from build123d import *

# Parameters (mm, degrees)
SKETCH021_R      = 1.65
EXTRUDE021_DEPTH = 5
EXTRUDE001_DEPTH = 4
FILLET003_R      = 0.5
BOX005_W         = 48
BOX005_H         = 47
BOX005_DEPTH     = 10
EXTRUDE037_DEPTH = 6
SKETCH038_W      = 10
SKETCH038_H      = 14.5
SKETCH038_R      = 1.25
EXTRUDE038_DEPTH = 4
SKETCH039_W      = 5
SKETCH039_H      = 16
SKETCH039_R      = 1.65
EXTRUDE039_DEPTH = 5
EXTRUDE040_DEPTH = 7
SKETCH020_R      = 1.65
SKETCH020_R_2    = 1.25
SKETCH020_W      = 45
SKETCH020_H      = 10
EXTRUDE036_DEPTH = 4


with BuildPart() as gpshold:
    # Sketch021 → Extrude021 (new body)
    with BuildSketch(Plane.XZ):
        Polygon((65, 28.5), (71, 28.5), (71, 2.5), (65, 2.5), (65, 9), (67, 9), (67, 22), (65, 22), align=None)
        with Locations((67.85, 25.7)):
            Circle(SKETCH021_R, mode=Mode.SUBTRACT)
        with Locations((67.85, 5.4)):
            Circle(SKETCH021_R, mode=Mode.SUBTRACT)
    extrude(amount=EXTRUDE021_DEPTH)


with BuildPart() as gpshold_1:
    # Extrude021 placement: moved
    add(gpshold.part.moved(Location((0, 78.75, 0))))


with BuildPart() as obj1:
    # Sketch001 → Extrude001 (new body)
    with BuildSketch(Plane.XY):
        with BuildLine():
            Line((19.03, 74.44), (19.03, 77.44))
            Line((19.03, 77.44), (13.53, 77.44))
            Line((13.53, 71.94), (13.53, 77.44))
            Line((16.53, 71.94), (13.53, 71.94))
            ThreePointArc((16.53, 71.94), (18.297767, 72.672233), (19.03, 74.44))
        make_face()
        with BuildLine():
            Line((60.53, 34.86), (55.03, 34.86))
            Line((55.03, 34.86), (55.03, 37.86))
            ThreePointArc((57.53, 40.36), (55.762233, 39.627767), (55.03, 37.86))
            Line((60.53, 40.36), (57.53, 40.36))
            Line((60.53, 34.86), (60.53, 40.36))
        make_face()
    extrude(amount=EXTRUDE001_DEPTH)


with BuildPart() as obj1_1:
    # Extrude001 placement: moved
    add(obj1.part.moved(Location((0, 0, 2))))

    # Fillet003
    fillet003_edges = [obj1_1.edges().sort_by_distance(p)[0] for p in [
        (57.78, 34.86, 6),
        (55.03, 36.36, 6),
        (55.762233, 39.627767, 6),
        (60.53, 40.36, 4),
        (59.03, 40.36, 6),
        (60.53, 37.61, 6),
        (18.297767, 72.672233, 6),
        (19.03, 77.44, 4),
        (19.03, 75.94, 6),
        (13.53, 77.44, 4),
        (16.28, 77.44, 6),
        (13.53, 71.94, 4),
        (13.53, 74.69, 6),
        (15.03, 71.94, 6),
    ]]
    fillet(fillet003_edges, radius=FILLET003_R)


with BuildPart() as obj1_2:
    # Fillet003 placement: moved
    add(obj1_1.part.moved(Location((0, 0, 13))))


with BuildPart() as obj2:
    # Box005 → Box005 (new body)
    with BuildSketch(Plane(origin=(13, 34, 15.25), x_dir=(1, 0, 0), z_dir=(0, 0, 1))):
        with Locations((24, 23.5)):
            Rectangle(BOX005_W, BOX005_H)
    extrude(amount=BOX005_DEPTH)


with BuildPart() as obj3:
    # Sketch037 → Extrude037 (new body)
    with BuildSketch(Plane.XY.offset(17)):
        with BuildLine():
            Line((3, 58.25), (13, 58.25))
            Line((13, 58.25), (13, 43.75))
            Line((13, 43.75), (3, 43.75))
            Line((3, 43.75), (3, 45.75))
            Line((3, 45.75), (6.5, 45.75))
            ThreePointArc((6.5, 45.75), (11.75, 51), (6.5, 56.25))
            Line((3, 56.25), (6.5, 56.25))
            Line((3, 58.25), (3, 56.25))
        make_face()
    extrude(amount=EXTRUDE037_DEPTH)


with BuildPart() as obj3_1:
    # Extrude037 placement: moved
    add(obj3.part.moved(Location((0, 0, -4))))


with BuildPart() as obj4:
    # Sketch038 → Extrude038 (new body)
    with BuildSketch(Plane.XY.offset(17)):
        with Locations((8, 51)):
            Rectangle(SKETCH038_W, SKETCH038_H)
        with Locations((6.5, 51)):
            Circle(SKETCH038_R, mode=Mode.SUBTRACT)
    extrude(amount=EXTRUDE038_DEPTH)


with BuildPart() as obj4_1:
    # Extrude038 placement: moved
    add(obj4.part.moved(Location((0, 0, 1.5))))


with BuildPart() as obj5:
    # Sketch039 → Extrude039 (new body)
    with BuildSketch(Plane.XZ.offset(-78.75)):
        with Locations((10.25, 21)):
            Rectangle(SKETCH039_W, SKETCH039_H)
        with Locations((10.35, 26.35)):
            Circle(SKETCH039_R, mode=Mode.SUBTRACT)
    extrude(amount=EXTRUDE039_DEPTH)


with BuildPart() as obj6:
    # Sketch040 → Extrude040 (new body)
    with BuildSketch(Plane.XZ.offset(-78.75)):
        with BuildLine():
            ThreePointArc((11.321071, 13.05), (10.34, 14.8), (9.358929, 13.05))
            Line((9.358929, 13.05), (11.321071, 13.05))
        make_face()
        with BuildLine():
            ThreePointArc((31.651071, 13.05), (30.67, 14.8), (29.688929, 13.05))
            Line((29.688929, 13.05), (31.651071, 13.05))
        make_face()
    extrude(amount=EXTRUDE040_DEPTH)


with BuildPart() as obj6_1:
    # Extrude040 placement: moved
    add(obj6.part.moved(Location((0, 7, 0))))


with BuildPart() as sensorhold005:
    # Sketch020 → Extrude036 (new body)
    with BuildSketch(Plane.XY):
        with BuildLine():
            Line((71, 78.75), (71, 60))
            Line((61, 60), (71, 60))
            Line((61, 34.75), (61, 60))
            Line((61, 34.75), (61, 60))
            Line((61, 34.75), (61, 60))
            Line((54.5, 34.75), (61, 34.75))
            ThreePointArc((54.5, 34.75), (48.202796, 49.952796), (33, 56.25))
            Line((3, 56.25), (33, 56.25))
            Line((3, 56.25), (3, 66.25))
            Line((3, 66.25), (7, 66.25))
            Line((7, 66.25), (7, 78.75))
            Line((7, 78.75), (34.55, 78.75))
            ThreePointArc((40.55, 78.75), (37.55, 80.878443), (34.55, 78.75))
            Line((40.55, 78.75), (71, 78.75))
        make_face()
        with Locations((5.55, 61.45)):
            Circle(SKETCH020_R, mode=Mode.SUBTRACT)
        with Locations((37.55, 77.7)):
            Circle(SKETCH020_R, mode=Mode.SUBTRACT)
        with Locations((65, 70)):
            Circle(SKETCH020_R_2, mode=Mode.SUBTRACT)
        with Locations((34.05, 66.45)):
            Rectangle(SKETCH020_W, SKETCH020_H, mode=Mode.SUBTRACT)
    extrude(amount=EXTRUDE036_DEPTH)


with BuildPart() as sensorhold005_1:
    # Extrude036 placement: moved
    add(sensorhold005.part.moved(Location((0, 0, 13))))

    # Fusion034: union obj3, obj4, obj5, obj6
    add(obj3_1.part)
    add(obj4_1.part)
    add(obj5.part)
    add(obj6_1.part)

    # Cut016: cut obj2
    add(obj2.part, mode=Mode.SUBTRACT)

    # Fusion035: union obj1
    add(obj1_2.part)

    # Fusion036: union gpsHold
    add(gpshold_1.part)


solid = sensorhold005_1.part
Model file for the job. Use its own axes, mm. A direction names the side the tool comes from. Give positions to 0.01 mm unless a question says otherwise; leave off trailing zeros. Order: outer loops, then holes, each group sorted by start corner. A loop starts at its lowest first (then second) coordinate and runs counter-clockwise, first axis right, second up. Notation, with made-up numbers: (3, 6) - (21, 6) arc R24 ccw to (21, 42) - close; hole circle Ø4 at (62.25, 54). An arc over 180 degrees is marked (long way). Write item = value, one per line. Start each with the question number.
1. Two-plate mould, pull along Z, no slides. Class faces 5 (the flat face through (67, 76, 19)), 6 (the cylindrical face through (9.99, 76.28, 24.74)), 7 (the flat face through (3, 55, 19)), 8 (the flat face through (42, 58, 15.25)): pulls with the +Z half, pulls with the -Z half, needs draft (parallel to the pull), parting line crosses it, or undercut.
2. Cut at D-D, the plane x = 21.5. List the corners of the cut face in (y, z).
3. Which spindle directions (+Z, -Z, +X, -X, +Y, -Y) get a long thin tool onto all of the face, cutting with end or side? Do faces 1 (the cylindrical face through (30.7, 82.3, 14.8)), 2 (the flat face through (19.03, 76, 17)), 3 (the flat face through (65, 76, 6)), 4 (the flat face through (58, 34.86, 17)). Say none if no direction does.
4. Cut at C-C, the plane x = 59. List the corners of the cut face in (y, z).
5. Drop flat-ended pins along their axis: P1, Ø1, axis at x = 5, z = 15.5, coming from the -Y side; P2, Ø0.8, axis at x = 14.5, z = 16.5, coming from the -Y side; P3, Ø2, axis at x = 10, y = 81, coming from the -Z side. Give the stop position or say it passes through.
6. Probe line 1 along X through (y, z) = (70, 13.9); line 2 along Y through (x, z) = (5.55, 14.9); line 3 along Z through (x, y) = (67.85, 76.7). List the from-to ranges inside material, lowest first.
7. Cut at A-A, the plane x = 30.67. List the corners of the cut face in (y, z), and give its area (3 significant figures).
8. Cut at B-B, the plane y = 51. List the corners of the cut face in (x, z), and give its area (3 significant figures).
Taken from the geometry:
q1.face_5 = undercut
q1.face_6 = undercut
q1.face_7 = needs draft
q1.face_8 = pulls with the +Z half
q2.outline = (56.25, 13) - (61.45, 13) - (61.45, 15.25) - (56.25, 15.25) - close; (71.45, 13) - (78.75, 13) - (78.75, 15.25) - (71.45, 15.25) - close
q3.face_1 = +Y
q3.face_2 = +Z, +Y, -Y
q3.face_3 = -Z, -X, +Y, -Y
q3.face_4 = +Z, +X, -X, -Y
q4.outline = (34.75, 13) - (78.75, 13) - (78.75, 15.25) - (40.36, 15.25) - (40.36, 18.5) arc R0.5 ccw to (39.86, 19) - (35.36, 19) arc R0.5 ccw to (34.86, 18.5) - (34.86, 15.25) - (34.75, 15.25) - close
q5.P1 = 43.75
q5.P2 = 71.94
q5.P3 = 13.05
q6.line_1 = 7 to 11.55, 56.55 to 63.75, 66.25 to 71
q6.line_2 = 43.75 to 45.75, 56.25 to 59.8, 63.1 to 66.25
q6.line_3 = 2.5 to 3.75, 7.05 to 24.05, 27.35 to 28.5
q7.outline = (56.25, 13) - (61.45, 13) - (61.45, 15.25) - (56.25, 15.25) - close; (71.45, 13) - (78.75, 13) - (78.75, 13.05) - (85.75, 13.05) - (85.75, 14.8) - (78.75, 14.8) - (78.75, 15.25) - (71.45, 15.25) - close
q7.area = 40.4 mm²
q8.outline = (3, 18.5) - (5.25, 18.5) - (5.25, 22.5) - (3, 22.5) - close; (7.75, 18.5) - (11.75, 18.5) - (11.75, 13) - (13, 13) - (13, 22.5) - (7.75, 22.5) - close; (47.08, 13) - (61, 13) - (61, 15.25) - (47.08, 15.25) - close
q8.area = 68.2 mm²
